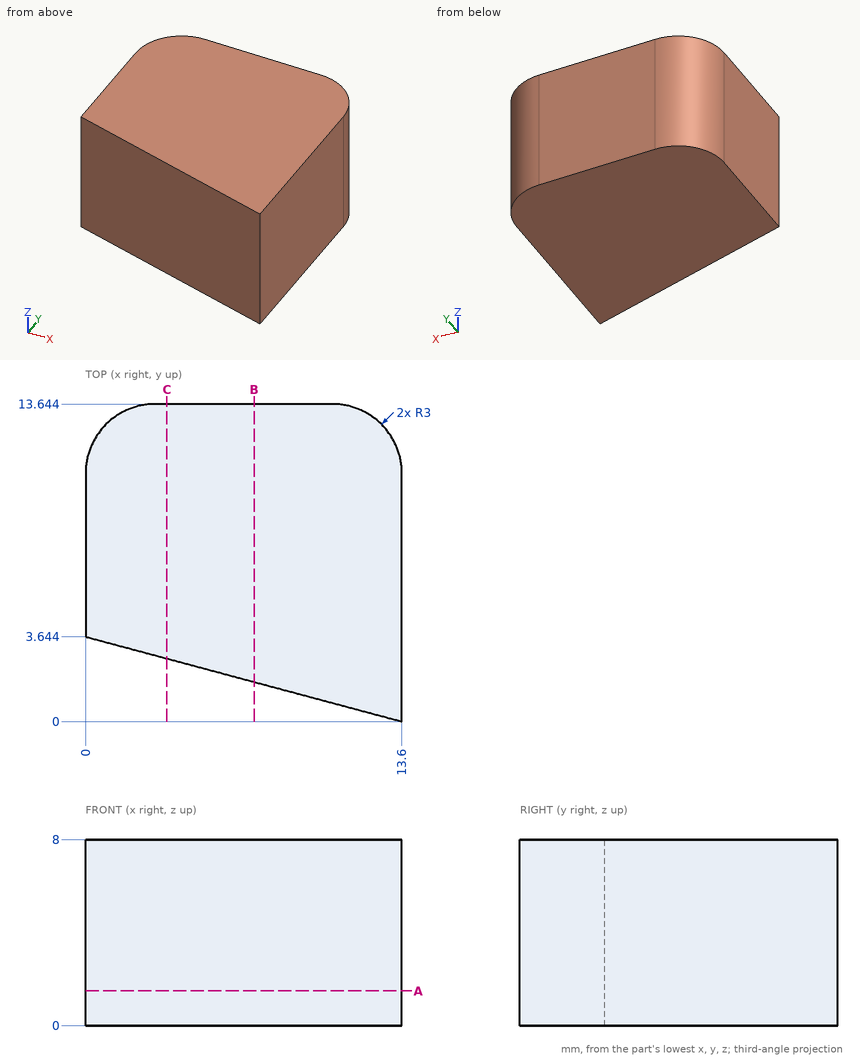
For this review, use the dimensioned drawing (mm, ordinates from the lowest corner) and the shaded views. Give positions to 0.01 mm unless a question says otherwise; leave off trailing zeros. Order: outer loops, then holes, each group sorted by start corner. A loop starts at its lowest first (then second) coordinate and runs counter-clockwise, first axis right, second up. Notation, with made-up numbers: M -33,19 L -26,19 A33 cw -26,50 Z; hole C 41,45 d4. An arc over 180 degrees is marked long. Use one line per item in the form item = value. Start each with the question number.
Item 1: We need section C-C on x = 3.5. Give the boundary of the cut face in (y, z), plus the area to 3 significant figures.
Item 2: To check wall thickness, follow line 1 along Y through (x, z) = (4, 5); line 2 along Y through (x, z) = (4.5, 4.75); line 3 along X through (y, z) = (12.5, 3.5). State the ranges of each line that lie inside material, in increasing order. Write a range as from..to.
Item 3: We need section A-A on z = 1.5. Give the boundary of the cut face in (x, y), plus the area to 3 significant figures.
Item 4: We need section B-B on x = 7.25. Give the boundary of the cut face in (y, z).
Completed:
q1.outline = M 2.71,0 L 13.64,0 L 13.64,8 L 2.71,8 Z
q1.area = 87.5 mm²
q2.line_1 = 2.57..13.64
q2.line_2 = 2.44..13.64
q2.line_3 = 0.64..12.96
q3.outline = M 0,3.64 L 13.6,0 L 13.6,10.64 A3 ccw 10.6,13.64 L 3,13.64 A3 ccw 0,10.64 Z
q3.area = 157 mm²
q4.outline = M 1.7,0 L 13.64,0 L 13.64,8 L 1.7,8 Z
